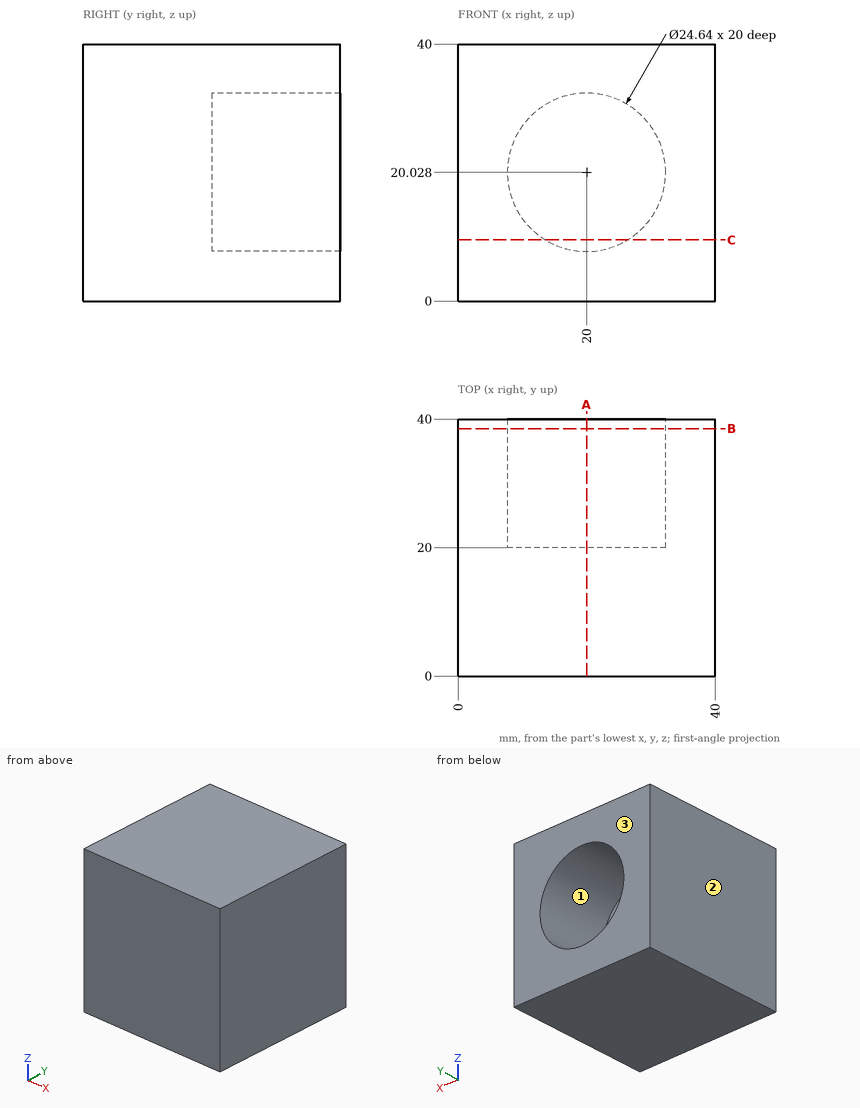
Study the drawing (mm; zero at the part's minimum x, y, z) and answer. Give positions to 0.01 mm unless a question says otherwise; leave off trailing zeros. Order: outer loops, then holes, each group sorted by start corner. A loop starts at its lowest first (then second) coordinate and runs counter-clockwise, first axis right, second up.
1. Section B-B, the plane y = 38.5 is taken. Determine the outline of the cut face in (x, z).
Result sheet:
outline: (0, 0) - (40, 0) - (40, 40) - (0, 40) - close; hole circle Ø24.64 at (20, 20.03)
2. Section A-A, the plane x = 20 is taken. Determine the outline of the cut face in (y, z), and give its area (3 significant figures).
Result sheet:
outline: (0, 0) - (40, 0) - (40, 7.71) - (20, 7.71) - (20, 32.35) - (40, 32.35) - (40, 40) - (0, 40) - close
area: 1,110 mm2
3. The mould has two halves that part along X. Classify the marked faces 1, 2 and 3: released by +X, released by -X, zero draft, split by the parting line, or undercut.
Result sheet:
face 1: undercut
face 2: released by -X
face 3: zero draft
4. This flat-tipped pin is pushed along its axis until it touches: P1, Ø15, axis at x = 20, z = 20.03, coming from the +Y side. Where does it stop, or does it pass through?
Result sheet:
P1: stops at y = 20
5. Section C-C, the plane z = 9.5 is taken. Determine the outline of the cut face in (x, y).
Result sheet:
outline: (0, 0) - (40, 0) - (40, 40) - (26.4, 40) - (26.4, 20) - (13.6, 20) - (13.6, 40) - (0, 40) - close
6. Straight lines are drawn through the part: L1, parallel to X at y = 29, z = 20; L2, parallel to Z at x = 20, y = 27; L3, parallel to Y at x = 25, z = 22.5. For each, find the intervals that lie inside material, in ascending order.
Result sheet:
L1: x = 0 to 7.68, 32.32 to 40
L2: z = 0 to 7.71, 32.35 to 40
L3: y = 0 to 20
